Geometry: final body of the model. Coordinates: model frame, mm. Round coordinates to 2 decimals unless told otherwise and drop trailing zeros. Loops run counter-clockwise (first coordinate to the right, second up) from the corner with the lowest first, then second, coordinate; pieces in that order, holes last. Notation, with made-up numbers: (58.5, -36.75) -> (93.5, -36.75) arc R19 cw to (93.5, -10.75) -> close; hole circle Ø5 at (65.5, 66). An arc over 180 degrees is marked (long way). Answer in a Markdown table with one row per item.
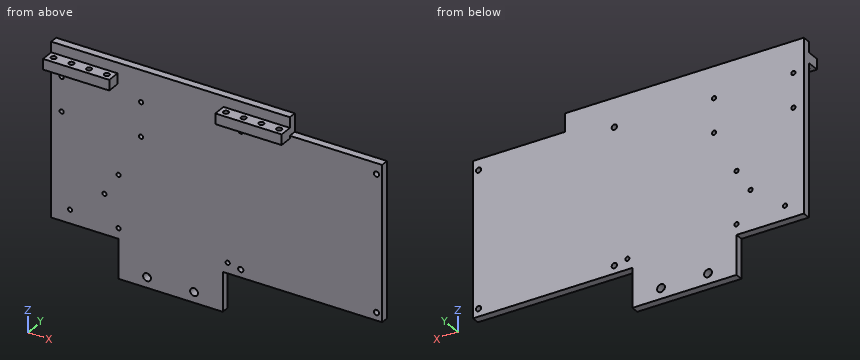
```python
from build123d import *

# Parameters (mm, degrees)
SKETCH1_W           = 116.078
SKETCH1_H           = 102.87
BOSS_EXTRUDE1_DEPTH = 3.81
SKETCH2_R           = 1.905
SKETCH2_W           = 32.766
SKETCH2_H           = 19.05
SKETCH2_W_2         = 32.639
CUT_EXTRUDE1_DEPTH  = 3.81
SKETCH3_W           = 32.258
SKETCH3_H           = 5.08
BOSS_EXTRUDE2_DEPTH = 6.35
SKETCH4_R           = 1.27
CUT_EXTRUDE2_DEPTH  = 5.08
SKETCH5_R           = 1.016
CUT_EXTRUDE4_DEPTH  = 3.81
SKETCH6_W           = 70
SKETCH6_H           = 75
BOSS_EXTRUDE3_DEPTH = 3.81
SKETCH7_R           = 1.27
CUT_EXTRUDE5_DEPTH  = 3.81


with BuildPart() as part:
    # Sketch1 → Boss-Extrude1 (new body)
    with BuildSketch(Plane(origin=(0, 0, 0), x_dir=(1, 0, 0), z_dir=(0, 1, 0))):
        with Locations((58.039, 51.435)):
            Rectangle(SKETCH1_W, SKETCH1_H)
    extrude(amount=BOSS_EXTRUDE1_DEPTH)

    # Sketch2 → Cut-Extrude1 (cut)
    with BuildSketch(Plane(origin=(0, 3.81, 0), x_dir=(1, 0, 0), z_dir=(0, 1, 0))):
        with Locations(Location((46.609, 97.79, 0), (0, 0, 270))):
            Circle(SKETCH2_R)
        with Locations(Location((69.469, 97.79, 0), (0, 0, 270))):
            Circle(SKETCH2_R)
        with Locations((16.383, 93.345)):
            Rectangle(SKETCH2_W, SKETCH2_H)
        with Locations((99.7585, 93.345)):
            Rectangle(SKETCH2_W_2, SKETCH2_H)
    extrude(amount=-CUT_EXTRUDE1_DEPTH, mode=Mode.SUBTRACT)

    # Sketch3 → Boss-Extrude2 (add)
    with BuildSketch(Plane.XZ):
        with Locations((16.129, -7.62)):
            Rectangle(SKETCH3_W, SKETCH3_H)
        with Locations((99.949, -7.62)):
            Rectangle(SKETCH3_W, SKETCH3_H)
    extrude(amount=BOSS_EXTRUDE2_DEPTH)

    # Sketch4 → Cut-Extrude2 (cut)
    with BuildSketch(Plane.XY.offset(-5.08)):
        with Locations((3.175, -3.175)):
            Circle(SKETCH4_R)
        with Locations((11.811, -3.175)):
            Circle(SKETCH4_R)
        with Locations((20.447, -3.175)):
            Circle(SKETCH4_R)
        with Locations((29.083, -3.175)):
            Circle(SKETCH4_R)
        with Locations((86.995, -3.175)):
            Circle(SKETCH4_R)
        with Locations((95.631, -3.175)):
            Circle(SKETCH4_R)
        with Locations((104.267, -3.175)):
            Circle(SKETCH4_R)
        with Locations((112.903, -3.175)):
            Circle(SKETCH4_R)
    extrude(amount=-CUT_EXTRUDE2_DEPTH, mode=Mode.SUBTRACT)

    # Sketch5 → Cut-Extrude4 (cut)
    with BuildSketch(Plane(origin=(0, 3.81, 0), x_dir=(1, 0, 0), z_dir=(0, 1, 0))):
        with Locations(Location((25.908, 64.516, 0), (0, 0, 270))):
            Circle(SKETCH5_R)
        with Locations(Location((9.144, 77.216, 0), (0, 0, 270))):
            Circle(SKETCH5_R)
        with Locations(Location((32.766, 78.74, 0), (0, 0, 270))):
            Circle(SKETCH5_R)
        with Locations(Location((85.852, 78.74, 0), (0, 0, 270))):
            Circle(SKETCH5_R)
        with Locations(Location((32.766, 53.34, 0), (0, 0, 270))):
            Circle(SKETCH5_R)
        with Locations(Location((5.08, 31.75, 0), (0, 0, 270))):
            Circle(SKETCH5_R)
        with Locations(Location((43.688, 31.75, 0), (0, 0, 270))):
            Circle(SKETCH5_R)
        with Locations(Location((5.08, 15.24, 0), (0, 0, 270))):
            Circle(SKETCH5_R)
        with Locations(Location((43.688, 15.24, 0), (0, 0, 270))):
            Circle(SKETCH5_R)
    extrude(amount=-CUT_EXTRUDE4_DEPTH, mode=Mode.SUBTRACT)

    # Sketch6 → Boss-Extrude3 (add)
    with BuildSketch(Plane(origin=(0, 3.81, 0), x_dir=(1, 0, 0), z_dir=(0, 1, 0))):
        with Locations((125.932, 46.32)):
            Rectangle(SKETCH6_W, SKETCH6_H)
    extrude(amount=-BOSS_EXTRUDE3_DEPTH)

    # Sketch7 → Cut-Extrude5 (cut)
    with BuildSketch(Plane(origin=(0, 3.81, 0), x_dir=(1, 0, 0), z_dir=(0, 1, 0))):
        with Locations(Location((92.202, 14.01, 0), (0, 0, 270))):
            Circle(SKETCH7_R)
        with Locations(Location((92.202, 80.01, 0), (0, 0, 270))):
            Circle(SKETCH7_R)
        with Locations(Location((158.202, 80.01, 0), (0, 0, 270))):
            Circle(SKETCH7_R)
        with Locations(Location((158.202, 14.01, 0), (0, 0, 270))):
            Circle(SKETCH7_R)
    extrude(amount=-CUT_EXTRUDE5_DEPTH, mode=Mode.SUBTRACT)


solid = part.part
```
Item 1: Cut plane A-A (y = 2.25). Count the separate pieces of the cut face and the enclosed holes in it, then the cut area to 3 significant figures.
Answer:
| item | result |
|---|---|
| separate pieces | 1 |
| enclosed holes | 15 |
| area | 14,000 mm² |
Item 2: Pin query (flat end, axial travel): pin 1 Ø3.5 at (x, z) = (92.202, -80.01) entering from +Y; pin 2 Ø10 at (x, z) = (117, -74.5) entering from -Y; pin 3 Ø1.9 at (x, y) = (8.5, -3.5) entering from +Z; pin 4 Ø1.2 at (x, z) = (43.688, -31.75) entering from -Y. Return the tip coordinate at first contact, or that it passes through.
Answer:
| item | result |
|---|---|
| pin 1 | stops at y = 3.81 |
| pin 2 | stops at y = 0 |
| pin 3 | stops at z = -5.08 |
| pin 4 | passes through |
Item 3: Line query: probe 1 along X at (y, z) = (2, -97.79); probe 2 along X at (y, z) = (2, -80.01); probe 3 along Z at (x, y) = (27, 1.75). Output: solid intervals per line, ascending. Write a range as [from, to].
Answer:
| item | result |
|---|---|
| probe 1 | x = [32.77, 44.7], [48.51, 67.56], [71.37, 83.44] |
| probe 2 | x = [0, 90.93], [93.47, 156.93], [159.47, 160.93] |
| probe 3 | z = [-83.82, 0] |
Item 4: Cut plane B-B (x = 40.5). Output: boundary loops of the cut face in (y, z), then the cut area to 3 significant figures.
Answer:
| item | result |
|---|---|
| outline | (0, -102.87) -> (3.81, -102.87) -> (3.81, 0) -> (0, 0) -> close |
| area | 392 mm² |
Item 5: Cut plane C-C (z = -48.5). Output: boundary loops of the cut face in (x, y), then the cut area to 3 significant figures.
Answer:
| item | result |
|---|---|
| outline | (0, 0) -> (160.93, 0) -> (160.93, 3.81) -> (0, 3.81) -> close |
| area | 613 mm² |
